Can you work these out from the drawing? Everything is in mm from the part's minimum corner. A direction names the side the tool comes from. Coordinates: 2 decimals unless noted, no trailing zeros. Order: outer loops, then holes, each group sorted by start corner. A loop starts at its lowest first (then second) coordinate and runs counter-clockwise, first axis right, second up. Notation, with made-up numbers: (89.5, 27.25) -> (127.5, 27.25) arc R11 cw to (127.5, 42.25) -> close; hole circle Ø4 at (-35, 46.25). An arc over 180 degrees is marked (long way). Put each result on its own line as item: value. Start each with the question number.
Q1. If we section it at C-C (x = 37): Please give me the cut outline in (y, z).
Q2. Will these pins go through, and if not, where does the flat tip stop? pin 1 (6 mm diameter, centred on x = 21.5, z = 22.5, fed in from -Y) (1 decimal); pin 2 (8 mm diameter, centred on x = 24.5, z = 67, fed in from +Y); pin 3 (8 mm diameter, centred on x = 8, z = 54.5, fed in from -Y).
Q3. If we section it at B-B (y = 66): Please give me the cut outline in (x, z).
Q4. For the marked faces 1 and 2, which set-ups out of +Z, -Z, +X, -X, +Y, -Y let a thin tool reach every point of the face, with its end or its side?
Q5. Please list where these lines run through material, in increasing order: line 1 along X through (y, z) = (195, 26); line 2 along Y through (x, z) = (12, 48.5); line 3 along Y through (x, z) = (13.5, 18.5) (1 decimal).
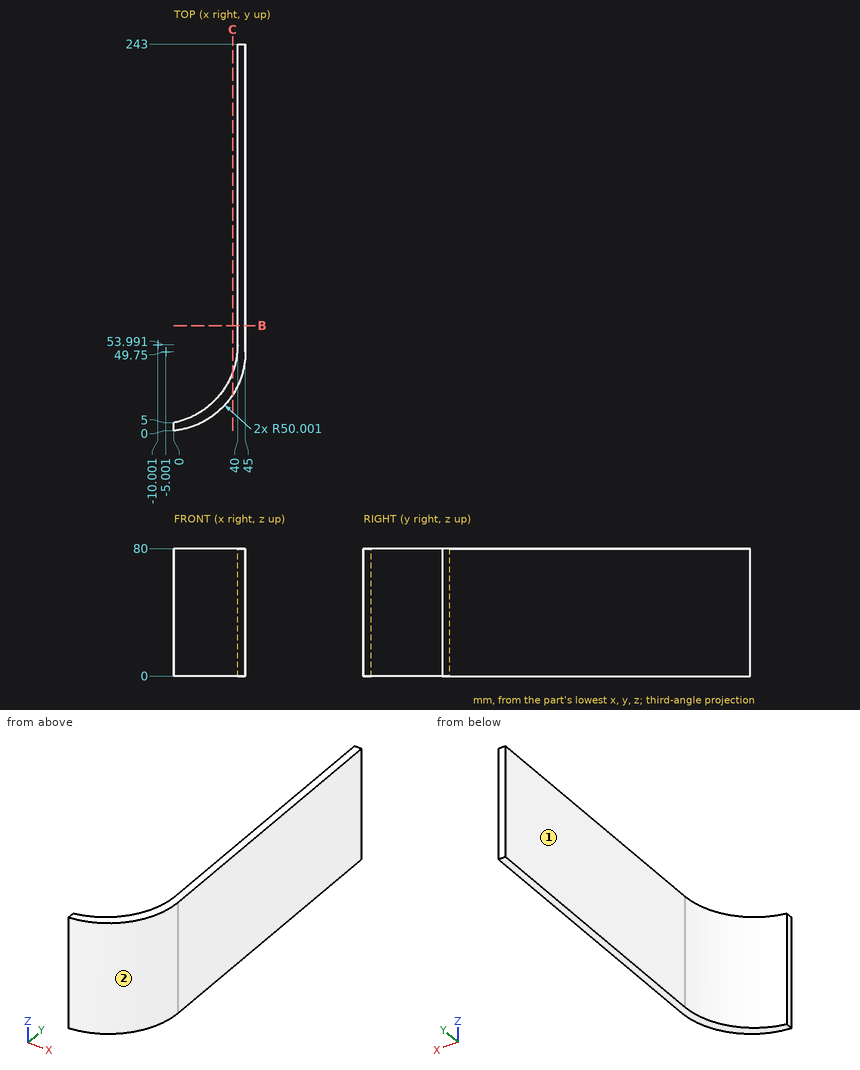
The answers:
1. outline: (22.62, 0) -> (36.93, 0) -> (36.93, 80) -> (22.62, 80) -> close
2. pin 1: y = 5.6
2. pin 2: y = 22.09
2. pin 3: y = 0.57
3. outline: (40, 0) -> (45, 0) -> (45, 80) -> (40, 80) -> close
4. face 1: +Z, -Z, -X, +Y
4. face 2: +Z, -Z, +X, -Y
5. line 1: 40 to 45
5. line 2: 2.73 to 9.09
5. line 3: 3.3 to 9.9
